```python
from build123d import *

# Parameters (mm, degrees)
EXTRUDE_1_DEPTH         = 17.5
SKETCH_3_R              = 23.5
CUT_EXTRUDE_1_DEPTH     = 9
HOLE_WIZARD_M14_1_D     = 12
HOLE_WIZARD_M14_1_DEPTH = 20
HOLE_WIZARD_M14_1_TIP   = 3.605163714
HOLE_WIZARD_M6_1_D      = 5
HOLE_WIZARD_M6_1_DEPTH  = 15
HOLE_WIZARD_M6_1_TIP    = 1.502151548
SKETCH_8_R              = 2.5
CUT_EXTRUDE_2_DEPTH     = 77.871280236


with BuildPart() as part:
    # 草图2 → 凸台-拉伸1 (new, symmetric)
    with BuildSketch(Plane.XY):
        with BuildLine():
            Line((0, 0), (0, -20))
            Line((0, -20), (20, -40))
            Line((20, -40), (80, -40))
            Line((80, -40), (100, -20))
            Line((100, -20), (100, 0))
            Line((100, 0), (71.5, 0))
            ThreePointArc((71.5, 0), (50, -21.500002185), (28.5, 0))
            Line((28.5, 0), (0, 0))
        make_face()
    extrude(amount=EXTRUDE_1_DEPTH, both=True)

    # 草图3 → 切除-拉伸1 (cut, symmetric)
    with BuildSketch(Plane.XY):
        with Locations((50, -2.185e-06)):
            Circle(SKETCH_3_R)
    extrude(amount=CUT_EXTRUDE_1_DEPTH, both=True, mode=Mode.SUBTRACT)

    # M14 螺纹孔1
    with Locations(Plane(origin=(0, 0, 0), x_dir=(1, 0, 0), z_dir=(0, 1, 0))):
        with Locations((15, 0), (85, 0)):
            Hole(HOLE_WIZARD_M14_1_D / 2, depth=HOLE_WIZARD_M14_1_DEPTH)
            with Locations((0, 0, -(HOLE_WIZARD_M14_1_DEPTH + HOLE_WIZARD_M14_1_TIP / 2))):  # 118° drill point
                Cone(0, HOLE_WIZARD_M14_1_D / 2, HOLE_WIZARD_M14_1_TIP, mode=Mode.SUBTRACT)

    # M6 螺纹孔1
    with Locations(Plane(origin=(60, -60, 0), x_dir=(-0.7071067811865476, -0.7071067811865476, 0), z_dir=(0.7071067811865476, -0.7071067811865476, 0))):
        with Locations((-33.284271247, 0)):
            Hole(HOLE_WIZARD_M6_1_D / 2, depth=HOLE_WIZARD_M6_1_DEPTH)
            with Locations((0, 0, -(HOLE_WIZARD_M6_1_DEPTH + HOLE_WIZARD_M6_1_TIP / 2))):  # 118° drill point
                Cone(0, HOLE_WIZARD_M6_1_D / 2, HOLE_WIZARD_M6_1_TIP, mode=Mode.SUBTRACT)

    # 草图8 → 切除-拉伸2 (cut, through all)
    with BuildSketch(Plane(origin=(52.928932188, -52.928932188, 0), x_dir=(-0.7071067811865476, -0.7071067811865476, 0), z_dir=(0.7071067811865476, -0.7071067811865476, 0))):
        with Locations(Location((-33.284271247, 0, 0), (0, 0, 180))):
            Circle(SKETCH_8_R)
    extrude(amount=-CUT_EXTRUDE_2_DEPTH, mode=Mode.SUBTRACT)


solid = part.part
```
Input: part model. Units: mm. Frame: model coordinates. A direction names the side the tool comes from. Coordinates: 2 decimals unless noted, no trailing zeros. Write each loop counter-clockwise with the first axis right and the second up, starting at its lowest first coordinate (ties: lowest second). Pieces come first, ordered by that corner, then holes. Notation, with made-up numbers: (71.5, 43.25) -> (89.5, 43.25) arc R6 cw to (89.5, 47.25) -> close; hole circle Ø9 at (3.5, 4.25). An arc over 180 degrees is marked (long way). Answer as a JSON object with one key per item and string values.
1. First-contact query: P1, Ø7, axis at x = 60.5, y = -10, coming from the +Z side; P2, Ø6, axis at y = -25, z = 3.5, coming from the -X side; P3, Ø9.5, axis at x = 15, z = 0, coming from the +Y side. Flat tips, straight axial feed; report the tip coordinate or a pass-through.
Result set:
{"P1": "passes through", "P2": "stops at x = 2", "P3": "stops at y = -20.75"}
2. Section A-A on y = -2.5. Return the cut outline in (x, z), then the cut area to 3 significant figures.
Result set:
{"outline": "(0, -17.5) -> (28.65, -17.5) -> (28.65, -9) -> (26.63, -9) -> (26.63, 9) -> (28.65, 9) -> (28.65, 17.5) -> (0, 17.5) -> close; (71.35, -17.5) -> (100, -17.5) -> (100, 17.5) -> (71.35, 17.5) -> (71.35, 9) -> (73.37, 9) -> (73.37, -9) -> (71.35, -9) -> close; hole circle Ø12 at (15, 0); hole circle Ø12 at (85, 0)", "area": "1,710 mm2"}
3. Section B-B on x = 50. Return the cut outline in (y, z).
Result set:
{"outline": "(-40, -17.5) -> (-21.5, -17.5) -> (-21.5, -9) -> (-23.5, -9) -> (-23.5, 9) -> (-21.5, 9) -> (-21.5, 17.5) -> (-40, 17.5) -> close"}
4. Material intervals for line 1 (X direction, y = -6, z = -1); line 2 (Z direction, x = 85, y = -12); line 3 (Z direction, x = 12.5, y = -11.5), sorted ascending. Write a range as from..to.
Result set:
{"line 1": "x = 0..9.08, 20.92..27.28, 72.72..79.08, 90.92..100", "line 2": "z = -17.5..-6, 6..17.5", "line 3": "z = -17.5..-5.45, 5.45..17.5"}
5. Section D-D on y = -18. Count the separate pieces of the cut face and the enclosed holes in it, then the cut area to 3 significant figures.
Result set:
{"separate pieces": "2", "enclosed holes": "2", "area": "2,320 mm2"}
6. Access query for faces 1 (the face through (9.46, -10.14, 2.3)), 2 (the face through (49, -24, -17.5)). Directions: +Z, -Z, +X, -X, +Y, -Y. A direction counts if a zero-diameter tool reaches every point of the face in a straight line with its end or side. Return the directions, or none.
Result set:
{"face 1": "+Y", "face 2": "-Z, +X, -X, +Y, -Y"}
7. Section C-C on z = -14. Return the cut outline in (x, y).
Result set:
{"outline": "(0, -20) -> (20, -40) -> (80, -40) -> (100, -20) -> (100, 0) -> (71.5, 0) arc R21.5 cw to (28.5, 0) -> (0, 0) -> close"}
8. Mould query, pull axis Y, two halves, no side actions, for faces 3 (the face through (50, -22, -9)), 4 (the face through (15.96, -22.98, 0.4)), 5 (the face through (72.29, -28.75, -0.11)). Classes: released by +Y, released by -Y, zero draft, split by the parting line, or undercut.
Result set:
{"face 3": "zero draft", "face 4": "released by +Y", "face 5": "undercut"}
